Part model, mm, in its own coordinate system. A direction names the side the tool comes from. Give positions to 0.01 mm unless a question says otherwise; leave off trailing zeros. Answer in a Markdown table with one row per item.
Autodesk Inventor part; units mm, degrees
ref_plane "YZ Plane" through (0, 0, 0) normal (1, 0, 0) x (0, 1, 0)
ref_plane "XZ Plane" through (0, 0, 0) normal (0, 1, 0) x (-1, 0, 0)
ref_plane "XY Plane" through (0, 0, 0) normal (0, 0, 1) x (1, 0, 0)
sketch "Sketch1" plane through (0, 0, 0) normal (0, 0, 1) x (1, 0, 0)
  circle A0 centre (-4064, 0) radius 361.95
  circle A1 centre (-4064, 0) radius 412.75
  line L0 (0, -577.85) -> (0, 577.85)
  point P0 (0, 0)
  dimension "d0" = 723.9
  dimension "d1" = 825.5
  dimension "d2" = 4064
revolve "Revolution1" add sketch "Sketch1" angle 30 about axis through (0, -10, 0) along (0, 1, 0)
sketch "Sketch10" plane through (-4064, 0, 0) normal (0, 0, -1) x (-1, 0, 0)
  circle A0 centre (0, 0) radius 387.35
  circle A1 centre (0, 0) radius 412.75 construction
  point P0 (-4064, 0)
  dimension "d34" = 774.7
extrude "Extrusion9" cut sketch "Sketch10" against normal blind 12.7
sketch "Sketch11" plane through (-3519.5272, 0, 2032) normal (0.5, 0, 0.8660254) x (0.8660254, 0, -0.5)
  circle A0 centre (0, 0) radius 361.95
  circle A1 centre (0, 0) radius 387.096
  circle A2 centre (0, 0) radius 425.45
  line L0 (4064, -595.63) -> (4064, 595.63)
  point P0 (4064, 0)
  dimension "d37" = 774.192
  dimension "d38" = 850.9
extrude "Extrusion10" cut sketch "Sketch11" against normal blind 6.35 contours A2
extrude "Extrusion11" add sketch "Sketch11" along normal blind 6.35 contours A0 | A1
revolve "Revolution2" cut sketch "Sketch11" angle 0.5 about axis through (0, -10, 0) along (0, 1, 0) contours A0
fillet "Fillet3" radius 0.7937 2 edges at (-3857.9382, 0, 2220.047) (-3676.65, 0, 12.7)
chamfer "Chamfer3" distance 0.7937 angle 45 2 edges at (-3851.5872, 0, 2231.0473) (-3676.65, 0, 0)
properties part number "A1-19027-100-04 HCWI elbow - male" material "Iron, HCWI"
(1) Pull direction Y, two halves, no side cores. Call faces 3 (the face through (-3199.73, 116.27, 1847.46)), 4 (the face through (-3677.025, 17.031, 6.272)), 5 (the face through (-3815.29, -112.66, 2210.09)): +Y half, -Y half, draft (parallel to the pull), parting line (faces both ways), or undercut.
Recorded:
| item | result |
|---|---|
| face 3 | parting line |
| face 4 | undercut |
| face 5 | draft |
(2) Which spindle directions (+Z, -Z, +X, -X, +Y, -Y) get a long thin tool onto all of the face, cutting with end or side? Do faces 1 (the face through (-3760, -243, 0)), 2 (the face through (-3719, -113, 12.7)). Say none if no direction does.
Recorded:
| item | result |
|---|---|
| face 1 | -Z, +X, -X, +Y, -Y |
| face 2 | -Z |
(3) Pin check, flat tips, straight feed: pin 1 Ø5 at (x, z) = (-4121, 1437.5) entering from -Y; pin 2 Ø6 at (x, z) = (-4218, 1119) entering from +Y; pin 3 Ø10 at (y, z) = (170.5, 582) entering from +X. Stop position of each tip, or through.
Recorded:
| item | result |
|---|---|
| pin 1 | stops at y = -285.56 |
| pin 2 | stops at y = 286.72 |
| pin 3 | stops at x = -3639.5 |
(4) Drill centre lines: line 1 along Y through (x, z) = (-4064, 6.5); line 2 along Y through (x, z) = (-3428, 1549); line 3 along X through (y, z) = (148.5, 464.5). Where is each one in solid material? Low to high.
Recorded:
| item | result |
|---|---|
| line 1 | y = -412.75 to -387.35, 387.35 to 412.75 |
| line 2 | y = -281.06 to -199.09, 199.09 to 281.06 |
| line 3 | x = -4424.8 to -4369.46, -3704.91 to -3649.45 |
